Design review of the part built by this model. Coordinates are the model's own, in mm. Face numbers are marked on the shaded views. A direction names the side the tool comes from. Give positions to 0.01 mm unless a question says otherwise; leave off trailing zeros. Order: outer loops, then holes, each group sorted by start corner. A loop starts at its lowest first (then second) coordinate and runs counter-clockwise, first axis right, second up.
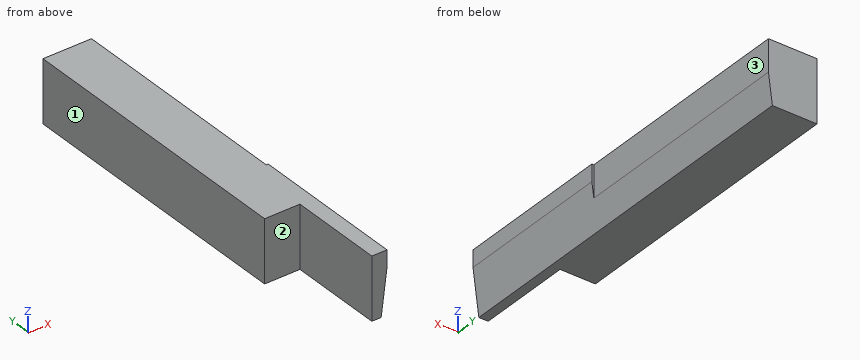
```python
from build123d import *

# Parameters (mm, degrees)
F0_W     = 25
F0_H     = 32
F1_DEPTH = 151
F2_W     = 6.8026450463
F2_H     = 32
F3_DEPTH = 49
F4_W     = 1
F4_H     = 32
F5_DEPTH = 81
F7_DEPTH = 248


with BuildPart() as f1:
    # F0 (on Front) → F1 (new body)
    with BuildSketch(Plane.XZ):
        with Locations((-12.5, -16)):
            Rectangle(F0_W, F0_H)
    extrude(amount=F1_DEPTH)

    # F2 (on face) → F3 (join)
    with BuildSketch(Plane.XZ.offset(151)):
        with Locations((-3.4013225231, -16)):
            Rectangle(F2_W, F2_H)
    extrude(amount=F3_DEPTH)

    # F4 (on face) → F5 (join)
    with BuildSketch(Plane.XZ.offset(200)):
        with Locations((0.5, -16)):
            Rectangle(F4_W, F4_H)
    extrude(amount=-F5_DEPTH)

    # F6 (on face) → F7 (cut)
    with BuildSketch(Plane(origin=(0, 0, 0), x_dir=(-1, 0, 0), z_dir=(0, 1, 0))):
        Polygon((2.8292152565, -38.3428484201), (-1.4198042918, -5.388750229), (-12.2544799853, -38.3428484201), align=None)
    extrude(amount=-F7_DEPTH, mode=Mode.SUBTRACT)


solid = f1.part
```
1. For pin 1 (18 mm diameter, centred on y = -69, z = -7, fed in from +X); pin 2 (0.8 mm diameter, centred on x = 0.5, z = -11, fed in from +Y); pin 3 (8 mm diameter, centred on y = -135, z = -17, fed in from +X); pin 4 (8 mm diameter, centred on x = -5, z = -18.5, fed in from +Y), all flat-tipped, find the tip position at first contact; note any pin that passes through.
Recorded:
pin 1: stops at x = 0
pin 2: stops at y = -119
pin 3: stops at x = 0.44
pin 4: stops at y = 0
2. Take a section at A-A (z = -5). State the section outline as (x, y) points, then the cut area to 3 significant figures.
Recorded:
outline: (-25, -151) - (-6.8, -151) - (-6.8, -200) - (1, -200) - (1, -119) - (0, -119) - (0, 0) - (-25, 0) - close
area: 4,190 mm2
3. Machinability: for the marked faces 1, 2 and 3, which of the approach directions +Z, -Z, +X, -X, +Y, -Y give a long, thin tool a straight path to every point of the face, cutting with its end or side? Answer none if there is none.
Recorded:
face 1: +Z, -Z, -X, +Y, -Y
face 2: +Z, -Z, -X, -Y
face 3: +Z, -Z, +X, +Y
4. Take a section at C-C (x = -22.75). State the section outline as (y, z) points.
Recorded:
outline: (-151, -32) - (0, -32) - (0, 0) - (-151, 0) - close
5. Take a section at D-D (z = -13.5). State the section outline as (x, y) points.
Recorded:
outline: (-25, -151) - (-6.8, -151) - (-6.8, -200) - (0.37, -200) - (0.37, -119) - (0, -119) - (0, 0) - (-25, 0) - close
6. For line 1 along Y through (x, z) = (-8.5, -10); line 2 along X through (y, z) = (-46, -7.5); line 3 along X through (y, z) = (-169, -3), list the stretches that pass through material, from the lowest coordinate up.
Recorded:
line 1: y = -151 to 0
line 2: x = -25 to 0
line 3: x = -6.8 to 1
7. Take a section at B-B (y = -23.5). State the section outline as (x, z) points.
Recorded:
outline: (-25, -32) - (-2.01, -32) - (0, -16.4) - (0, 0) - (-25, 0) - close
